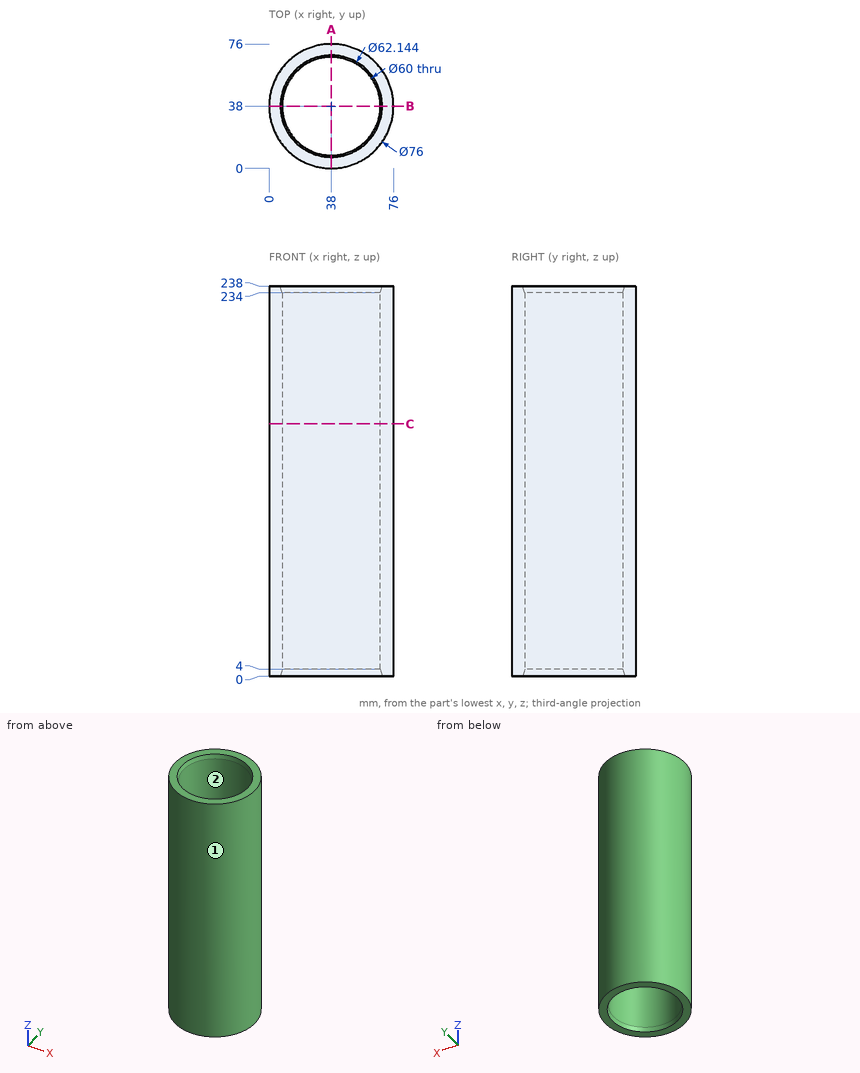
Study the drawing (mm; zero at the part's minimum x, y, z) and answer. Round coordinates to 2 decimals unless told otherwise and drop trailing zeros. Write each loop counter-clockwise with the first axis right and the second up, starting at its lowest first coordinate (ties: lowest second). Pieces come first, ordered by that corner, then holes. Notation, with made-up numbers: (73, 48.5) - (88, 48.5) arc R25 cw to (88, 62.5) - close; hole circle Ø3 at (39, 3). An arc over 180 degrees is marked (long way). Return JSON: item names as keys, results as strings. Group by question number.
Q1. Each of these flat-tipped pins is pushed along its axis until it touches: pin 1 Ø1.5 at (y, z) = (24, 88.5) entering from +X (1 decimal); pin 2 Ø1 at (y, z) = (11.5, 76) entering from -X; pin 3 Ø3 at (y, z) = (40, 58) entering from +X. Where does it stop, or does it pass through?
Q2. Find the intervals of material crossed by L1, parallel to Y at x = 38, z = 120; L2, parallel to X at y = 51, z = 67, in increasing order.
Q3. The part is cut by section C-C on z = 154. Write down the section's boundary in (x, y).
Q4. The mould has two halves that part along Y. Classify the marked faces 1 and 2: released by +Y, released by -Y, zero draft, split by the parting line, or undercut.
Q5. The part is cut by section A-A on x = 38. Write down the section's boundary in (y, z), then the cut area to 3 significant figures.
Solved:
{
 "1": {"pin 1": "x = 73.6", "pin 2": "x = 10.29", "pin 3": "x = 76"},
 "2": {"L1": "0 to 8, 68 to 76", "L2": "2.29 to 10.96, 65.04 to 73.71"},
 "3": {"outline": "circle Ø76 at (38, 38); hole circle Ø60 at (38, 38)"},
 "4": {"face 1": "split by the parting line", "face 2": "undercut"},
 "5": {"outline": "(0, 0) - (6.93, 0) - (8, 4) - (8, 234) - (6.93, 238) - (0, 238) - close; (68, 4) - (69.07, 0) - (76, 0) - (76, 238) - (69.07, 238) - (68, 234) - close", "area": "3,800 mm²"}
}
